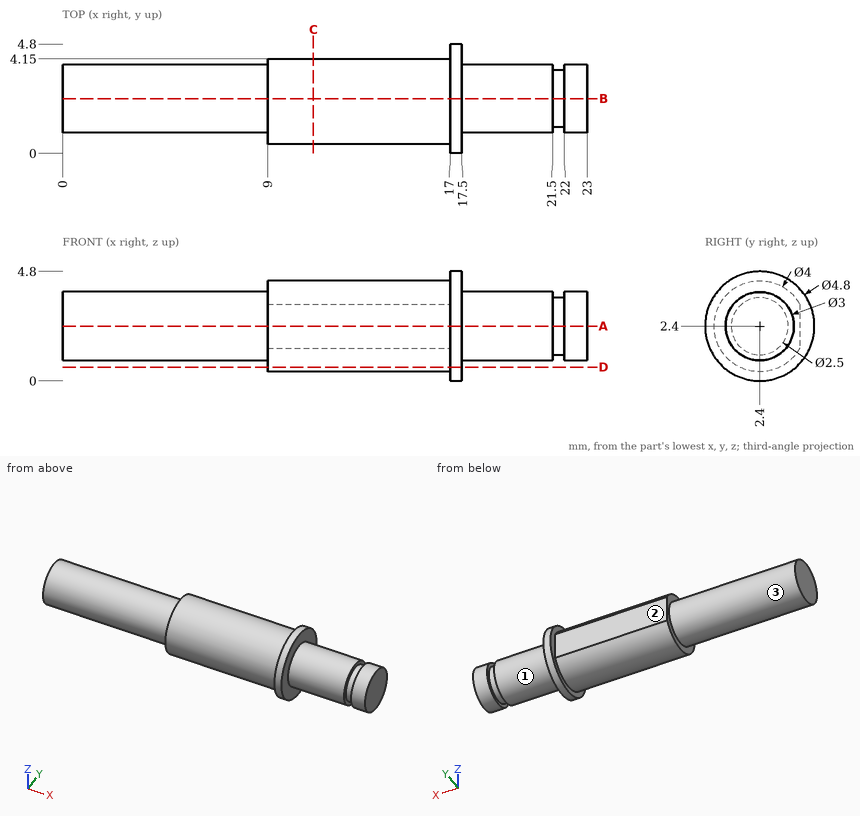
Study the drawing (mm; zero at the part's minimum x, y, z) and answer. A direction names the side the tool comes from. Give positions to 0.01 mm unless a question says otherwise; leave off trailing zeros. Order: outer loops, then holes, each group sorted by start corner. A loop starts at its lowest first (then second) coordinate and runs counter-clockwise, first axis right, second up. Notation, with made-up numbers: (-32.5, 64) -> (-26.5, 64) arc R24 ccw to (-26.5, 103) -> close; hole circle Ø4 at (79.5, -5.75). An arc over 180 degrees is marked (long way). Write item = value, one per line.
1. Given pin 1 (1 mm diameter, centred on x = 5.5, z = 2.5, fed in from -Y); pin 2 (1 mm diameter, centred on x = 4, y = 1.5, fed in from +Z); pin 3 (1 mm diameter, centred on x = 11, y = 3, fed in from -Z), each flat-ended and moving along its own axis, determine where each tip first touches the part or whether it passes through.
Numbers:
pin_1 = 0.9
pin_2 = 3.85
pin_3 = 0.4
2. For the marked faces 1, 2 and 3, determine the directions among +Z, -Z, +X, -X, +Y, -Y from which every point of the face is accessible in a straight line to the end or side of a thin tool.
Numbers:
face_1 = +X
face_2 = +Z, -Z, -X, +Y
face_3 = -X
3. A cutting plane is placed at D-D, the plane z = 0.6. Write down the section's boundary in (x, y).
Numbers:
outline = (9, 1.53) -> (17, 1.53) -> (17, 0.81) -> (17.5, 0.81) -> (17.5, 3.99) -> (17, 3.99) -> (17, 3.27) -> (9, 3.27) -> close
4. Straight lines are drawn through the part: line 1 along X through (y, z) = (2.1, 4.6); line 2 along X through (y, z) = (4.1, 1.6); line 3 along Z through (x, y) = (9.75, 2.45). For each, find the intervals that lie inside material, in ascending order.
Numbers:
line_1 = 17 to 17.5
line_2 = 9 to 17.5
line_3 = 0.4 to 4.4
5. A cutting plane is placed at C-C, the plane x = 11. Write down the section's boundary in (y, z), and give its area (3 significant figures).
Numbers:
outline = (4.15, 1.43) -> (4.15, 3.37) arc R2 ccw (long way) to start
area = 12.2 mm²
6. A cutting plane is placed at B-B, the plane y = 2.4. Write down the section's boundary in (x, z), and give its area (4 significant figures).
Numbers:
outline = (0, 0.9) -> (9, 0.9) -> (9, 0.4) -> (17, 0.4) -> (17, 0) -> (17.5, 0) -> (17.5, 0.9) -> (21.5, 0.9) -> (21.5, 1.15) -> (22, 1.15) -> (22, 0.9) -> (23, 0.9) -> (23, 3.9) -> (22, 3.9) -> (22, 3.65) -> (21.5, 3.65) -> (21.5, 3.9) -> (17.5, 3.9) -> (17.5, 4.8) -> (17, 4.8) -> (17, 4.4) -> (9, 4.4) -> (9, 3.9) -> (0, 3.9) -> close
area = 77.65 mm²
7. A cutting plane is placed at A-A, the plane z = 2.4. Write down the section's boundary in (x, y), and give its area (4 significant figures).
Numbers:
outline = (0, 0.9) -> (9, 0.9) -> (9, 0.4) -> (17, 0.4) -> (17, 0) -> (17.5, 0) -> (17.5, 0.9) -> (21.5, 0.9) -> (21.5, 1.15) -> (22, 1.15) -> (22, 0.9) -> (23, 0.9) -> (23, 3.9) -> (22, 3.9) -> (22, 3.65) -> (21.5, 3.65) -> (21.5, 3.9) -> (17.5, 3.9) -> (17.5, 4.8) -> (17, 4.8) -> (17, 4.15) -> (9, 4.15) -> (9, 3.9) -> (0, 3.9) -> close
area = 75.65 mm²
